Geometry: final body of the model. Coordinates: model frame, mm. A direction names the side the tool comes from. Coordinates: 2 decimals unless noted, no trailing zeros. Write each loop counter-clockwise with the first axis right and the second up, starting at its lowest first coordinate (ties: lowest second). Pieces come first, ordered by that corner, then holes. Notation, with made-up numbers: (83.5, 63.5) -> (90.5, 63.5) arc R27 ccw to (90.5, 97.5) -> close; hole circle Ø1 at (-37, -13.5). An arc over 180 degrees is marked (long way). One line per item, written item: value. Start each with the question number.
from build123d import *

# Parameters (mm, degrees)
SKETCH1_W           = 235
SKETCH1_H           = 22
BOSS_EXTRUDE1_DEPTH = 10
SKETCH2_W           = 235
SKETCH2_H           = 4.5
CUT_EXTRUDE1_DEPTH  = 6
CUT_EXTRUDE3_DEPTH  = 2.5
SKETCH9_R           = 1.5
CUT_EXTRUDE4_DEPTH  = 23
SKETCH_3_R          = 1.5
SKETCH_3_R_2        = 1.50188727
SKETCH_3_R_3        = 1.716965945
CUT_EXTRUDE_1_DEPTH = 23
CUT_EXTRUDE_2_DEPTH = 2
SKETCH_6_W          = 35
SKETCH_6_H          = 4.5
CUT_EXTRUDE_3_DEPTH = 5
SKETCH_9_W          = 3
SKETCH_9_H          = 22
CUT_EXTRUDE_4_DEPTH = 11


with BuildPart() as part:
    # Sketch1 → Boss-Extrude1 (new body)
    with BuildSketch(Plane(origin=(0, 0, 0), x_dir=(1, 0, 0), z_dir=(0, 1, 0))):
        Rectangle(SKETCH1_W, SKETCH1_H)
    extrude(amount=BOSS_EXTRUDE1_DEPTH)

    # Sketch2 → Cut-Extrude1 (cut)
    with BuildSketch(Plane(origin=(0, 10, 0), x_dir=(1, 0, 0), z_dir=(0, 1, 0))):
        with Locations((0, -4.700418011)):
            Rectangle(SKETCH2_W, SKETCH2_H)
        with Locations((0, 4.700418011)):
            Rectangle(SKETCH2_W, SKETCH2_H)
    extrude(amount=-CUT_EXTRUDE1_DEPTH, mode=Mode.SUBTRACT)

    # Sketch3 → Cut-Extrude3 (cut)
    with BuildSketch(Plane.XY.offset(11)):
        Polygon((-103.149147039, 6.25), (-104.736860279, 9), (-107.91228676, 9), (-109.5, 6.25), (-107.91228676, 3.5), (-104.736860279, 3.5), align=None)
        Polygon((-95.149147039, 6.25), (-93.561433799, 9), (-90.386007318, 9), (-88.798294078, 6.25), (-90.386007318, 3.5), (-93.561433799, 3.5), align=None)
        Polygon((-76.035154357, 9), (-79.210580838, 9), (-80.798294078, 6.25), (-79.210580838, 3.5), (-76.035154357, 3.5), (-74.447441117, 6.25), align=None)
        Polygon((-64.859727876, 3.5), (-66.447441117, 6.25), (-64.859727876, 9), (-61.684301396, 9), (-60.096588156, 6.25), (-61.684301396, 3.5), align=None)
        Polygon((-47.333448435, 9), (-50.508874915, 9), (-52.096588156, 6.25), (-50.508874915, 3.5), (-47.333448435, 3.5), (-45.745735195, 6.25), align=None)
        Polygon((-36.158021954, 3.5), (-37.745735195, 6.25), (-36.158021954, 9), (-32.982595474, 9), (-31.394882233, 6.25), (-32.982595474, 3.5), align=None)
        Polygon((-17.044029272, 6.25), (-18.631742513, 9), (-21.807168993, 9), (-23.394882233, 6.25), (-21.807168993, 3.5), (-18.631742513, 3.5), align=None)
        Polygon((-9.044029272, 6.25), (-7.456316032, 9), (-4.280889552, 9), (-2.693176311, 6.25), (-4.280889552, 3.5), (-7.456316032, 3.5), align=None)
        Polygon((10.06996341, 9), (6.894536929, 9), (5.306823689, 6.25), (6.894536929, 3.5), (10.06996341, 3.5), (11.65767665, 6.25), align=None)
        Polygon((21.24538989, 3.5), (19.65767665, 6.25), (21.24538989, 9), (24.420816371, 9), (26.008529611, 6.25), (24.420816371, 3.5), align=None)
        Polygon((38.771669332, 9), (35.596242851, 9), (34.008529611, 6.25), (35.596242851, 3.5), (38.771669332, 3.5), (40.359382572, 6.25), align=None)
        Polygon((49.947095812, 3.5), (48.359382572, 6.25), (49.947095812, 9), (53.122522293, 9), (54.710235533, 6.25), (53.122522293, 3.5), align=None)
        Polygon((69.061088494, 6.25), (67.473375254, 9), (64.297948773, 9), (62.710235533, 6.25), (64.297948773, 3.5), (67.473375254, 3.5), align=None)
        Polygon((77.061088494, 6.25), (78.648801734, 9), (81.824228215, 9), (83.411941455, 6.25), (81.824228215, 3.5), (78.648801734, 3.5), align=None)
    extrude(amount=-CUT_EXTRUDE3_DEPTH, mode=Mode.SUBTRACT)

    # Sketch9 → Cut-Extrude4 (cut, through all)
    with BuildSketch(Plane.XY.offset(11)):
        with Locations((-106.324573519, 6.25)):
            Circle(SKETCH9_R)
        with Locations((-91.973720558, 6.25)):
            Circle(SKETCH9_R)
        with Locations((-77.622867597, 6.25)):
            Circle(SKETCH9_R)
        with Locations((-63.272014636, 6.25)):
            Circle(SKETCH9_R)
        with Locations((-48.921161675, 6.25)):
            Circle(SKETCH9_R)
        with Locations((-34.570308714, 6.25)):
            Circle(SKETCH9_R)
        with Locations((-20.219455753, 6.25)):
            Circle(SKETCH9_R)
        with Locations((-5.868602792, 6.25)):
            Circle(SKETCH9_R)
        with Locations((8.482250169, 6.25)):
            Circle(SKETCH9_R)
        with Locations((22.83310313, 6.25)):
            Circle(SKETCH9_R)
        with Locations((37.183956091, 6.25)):
            Circle(SKETCH9_R)
        with Locations((51.534809052, 6.25)):
            Circle(SKETCH9_R)
        with Locations((65.885662014, 6.25)):
            Circle(SKETCH9_R)
        with Locations((80.236514975, 6.25)):
            Circle(SKETCH9_R)
    extrude(amount=-CUT_EXTRUDE4_DEPTH, mode=Mode.SUBTRACT)

    # 草图3 → 切除-拉伸1 (cut, through all)
    with BuildSketch(Plane.XY.offset(11)):
        with Locations((80.236514975, 6.25)):
            Circle(SKETCH_3_R)
        with Locations((94.586514975, 6.25)):
            Circle(SKETCH_3_R_2)
        with Locations((108.936514975, 6.25)):
            Circle(SKETCH_3_R_3)
        with Locations((65.885662014, 6.25)):
            Circle(SKETCH_3_R)
    extrude(amount=-CUT_EXTRUDE_1_DEPTH, mode=Mode.SUBTRACT)

    # 草图4 → 切除-拉伸2 (cut)
    with BuildSketch(Plane.XY.offset(11)):
        Polygon((81.824228215, 3.5), (83.411941455, 6.25), (81.824228215, 9), (78.648801734, 9), (77.061088494, 6.25), (78.648801734, 3.5), align=None)
        Polygon((97.761941455, 6.25), (96.174228215, 9), (92.998801734, 9), (91.411088494, 6.25), (92.998801734, 3.5), (96.174228215, 3.5), align=None)
        Polygon((112.111941455, 6.25), (110.524228215, 9), (107.348801734, 9), (105.761088494, 6.25), (107.348801734, 3.5), (110.524228215, 3.5), align=None)
    extrude(amount=-CUT_EXTRUDE_2_DEPTH, mode=Mode.SUBTRACT)

    # 草图6 → 切除-拉伸3 (cut, through all)
    with BuildSketch(Plane(origin=(0, 4, 0), x_dir=(1, 0, 0), z_dir=(0, 1, 0))):
        with Locations((100, -4.700418011)):
            Rectangle(SKETCH_6_W, SKETCH_6_H)
        with Locations((100, 4.700418011)):
            Rectangle(SKETCH_6_W, SKETCH_6_H)
        with Locations((-100, -4.700418011)):
            Rectangle(SKETCH_6_W, SKETCH_6_H)
        with Locations((-100, 4.700418011)):
            Rectangle(SKETCH_6_W, SKETCH_6_H)
    extrude(amount=-CUT_EXTRUDE_3_DEPTH, mode=Mode.SUBTRACT)

    # 草图9 → 切除-拉伸4 (cut, through all)
    with BuildSketch(Plane(origin=(0, 10, 0), x_dir=(1, 0, 0), z_dir=(0, 1, 0))):
        with Locations((-116, 0)):
            Rectangle(SKETCH_9_W, SKETCH_9_H)
    extrude(amount=-CUT_EXTRUDE_4_DEPTH, mode=Mode.SUBTRACT)


solid = part.part
Q1. Draft query along Z for faces 1 (the flat face through (-36, 8, 8.5)), 2 (the flat face through (0, 10, 9)), 3 (the flat face through (-1, 4, -5)). Return one class per face: pulls with the +Z half, pulls with the -Z half, needs draft (parallel to the pull), parting line crosses it, or undercut.
Q2. First-contact query: P1, Ø1.8, axis at x = 51.53, y = 6.25, coming from the -Z side; P2, Ø1.6, axis at x = 36, y = 7, coming from the +Z side; P3, Ø1.3, axis at x = 7, z = 4, coming from the +Y side; P4, Ø5, axis at x = 94.59, y = 6.25, coming from the +Z side. Flat tips, straight axial feed; report the tip coordinate or a pass-through.
Q3. Access query for faces 4 (the flat face through (-76, 7, 8.5)), 5 (the flat face through (-82.5, 2, -5)), 6 (the flat face through (82.5, 2, -5)), 7 (the flat face through (-1, 4, 5)). Directions: +Z, -Z, +X, -X, +Y, -Y. A direction counts if a zero-diameter tool reaches every point of the face in a straight line with its end or side. Return the directions, or none.
Q4. Cut plane C-C on x = -15. Output: boundary loops of the cut face in (y, z).
Q5. Line query: L1, parallel to Z at x = 12, y = 5; L2, parallel to Z at x = -18.5, y = 8; L3, parallel to Y at x = 42.5, z = -4. Output: solid intervals per line, ascending. Write a range as from..to.
Q6. Cut plane A-A on x = 101.5. Output: boundary loops of the cut face in (y, z), and give its area (3 significant figures).
Q7. Cut plane B-B on y = 1.75. Output: boundary loops of the cut face in (x, z).
Solution:
1. face 1: pulls with the +Z half
1. face 2: needs draft
1. face 3: undercut
2. P1: through
2. P2: z = 8.5
2. P3: y = 4
2. P4: z = 9
3. face 4: +Z
3. face 5: -X, +Y, -Y
3. face 6: +X, +Y, -Y
3. face 7: +X, -X, +Y
4. outline: (0, -11) -> (10, -11) -> (10, -6.95) -> (4, -6.95) -> (4, -2.45) -> (10, -2.45) -> (10, 2.45) -> (4, 2.45) -> (4, 6.95) -> (10, 6.95) -> (10, 11) -> (0, 11) -> close
5. L1: -11..-6.95, -2.45..2.45, 6.95..11
5. L2: -11..-6.95, -2.45..2.45, 6.95..8.5
5. L3: 0..4
6. outline: (0, -11) -> (10, -11) -> (10, -6.95) -> (0, -6.95) -> close; (0, -2.45) -> (10, -2.45) -> (10, 2.45) -> (0, 2.45) -> close; (0, 6.95) -> (10, 6.95) -> (10, 11) -> (0, 11) -> close
6. area: 130 mm²
7. outline: (-114.5, -11) -> (117.5, -11) -> (117.5, -6.95) -> (82.5, -6.95) -> (82.5, -2.45) -> (117.5, -2.45) -> (117.5, 2.45) -> (82.5, 2.45) -> (82.5, 6.95) -> (117.5, 6.95) -> (117.5, 11) -> (-114.5, 11) -> (-114.5, 6.95) -> (-82.5, 6.95) -> (-82.5, 2.45) -> (-114.5, 2.45) -> (-114.5, -2.45) -> (-82.5, -2.45) -> (-82.5, -6.95) -> (-114.5, -6.95) -> close
